Here's how the part is built. I have some questions about the finished solid (model axes, mm). A direction names the side the tool comes from. Give positions to 0.01 mm unless a question says otherwise; leave off trailing zeros. Write each loop counter-clockwise with the first axis right and the second up, starting at its lowest first coordinate (ties: lowest second). Pieces come first, ordered by that corner, then holes. Notation, with made-up numbers: (73, 52) - (103, 52) arc R28 ccw to (103, 81) - close; hole circle Ø8 at (15, -22). An arc over 180 degrees is marked (long way). One line per item, written item: value. Start each with the question number.
1) I'm going to push a flat-ended pin straight in: P1, Ø2, axis at y = 4, z = 0, coming from the +X side. Where does the tip first touch, or does it pass through?
2) Imagine slicing it at B-B on y = 7. Write out the boundary of the cut face in (x, z).
3) On a 3-axis mill with a long thin cutter (end or side, diameter ignored), from which of +Z, -Z, +X, -X, +Y, -Y can I reach the whole of each face in a straight line? I mean faces 5 (the cylindrical face through (5.449, -0.889, 27.445)), 6 (the flat face through (3, 63.5, -3)). Say none if no direction works.
4) Imagine slicing it at A-A on x = 30.5. Write out the boundary of the cut face in (y, z).
5) Imagine slicing it at D-D on z = -6.5. Write out the boundary of the cut face in (x, y).
6) Please list where these lines run through material, in increasing order: L1, parallel to X at y = -20, z = -10; L2, parallel to Z at x = 28, y = -10.5; L3, parallel to Z at x = 34, y = 14. Write a range as [from, to].
7) We'd pull the mould along Z, two halves only. Please class faces 1 (the flat face through (17, -1, 38.1)), 2 (the flat face through (20.9, -0.9, -31.1)), 3 (the flat face through (3, -63.5, -3)), 4 (the flat face through (16, -1, -38.1)): +Z half, -Z half, draft (parallel to the pull), parting line (faces both ways), or undercut.
8) Imagine slicing it at C-C on x = 14. Write out the boundary of the cut face in (y, z), plus the area to 3 significant figures.
from build123d import *

# Parameters (mm, degrees)
F1_DEPTH = 63.5


with BuildPart() as f1:
    # F0 (on Front) → F1 (new body, symmetric)
    with BuildSketch(Plane.XZ):
        with BuildLine():
            Line((0, 38.1), (0, 0))
            Line((0, 0), (0, -38.1))
            Line((0, -38.1), (33.02, -38.1))
            ThreePointArc((33.02, -38.1), (35.56, -35.56), (33.02, -33.02))
            Line((33.02, -33.02), (8.410474, -29.122234))
            ThreePointArc((8.410474, -29.122234), (5.480366, -27.481295), (4.318, -24.330563))
            Line((4.318, -24.330563), (4.318, 0))
            Line((4.318, 0), (4.318, 24.330563))
            ThreePointArc((4.318, 24.330563), (5.480366, 27.481295), (8.410474, 29.122234))
            Line((8.410474, 29.122234), (33.02, 33.02))
            ThreePointArc((33.02, 33.02), (35.56, 35.56), (33.02, 38.1))
            Line((33.02, 38.1), (0, 38.1))
        make_face()
    extrude(amount=F1_DEPTH, both=True)


solid = f1.part
Numbers:
1. P1: x = 4.32
2. outline: (0, -38.1) - (33.02, -38.1) arc R2.54 ccw to (33.02, -33.02) - (8.41, -29.12) arc R4.85 cw to (4.32, -24.33) - (4.32, 24.33) arc R4.85 cw to (8.41, 29.12) - (33.02, 33.02) arc R2.54 ccw to (33.02, 38.1) - (0, 38.1) - close
3. face 5: +X, +Y, -Y
3. face 6: +Z, -Z, +X, -X, +Y
4. outline: (-63.5, -38.1) - (63.5, -38.1) - (63.5, -32.62) - (-63.5, -32.62) - close; (-63.5, 32.62) - (63.5, 32.62) - (63.5, 38.1) - (-63.5, 38.1) - close
5. outline: (0, -63.5) - (4.32, -63.5) - (4.32, 63.5) - (0, 63.5) - close
6. L1: [0, 4.32]
6. L2: [-38.1, -32.22], [32.22, 38.1]
6. L3: [-37.9, -33.22], [33.22, 37.9]
7. face 1: +Z half
7. face 2: undercut
7. face 3: draft
7. face 4: -Z half
8. outline: (-63.5, -38.1) - (63.5, -38.1) - (63.5, -30.01) - (-63.5, -30.01) - close; (-63.5, 30.01) - (63.5, 30.01) - (63.5, 38.1) - (-63.5, 38.1) - close
8. area: 2,060 mm^2
